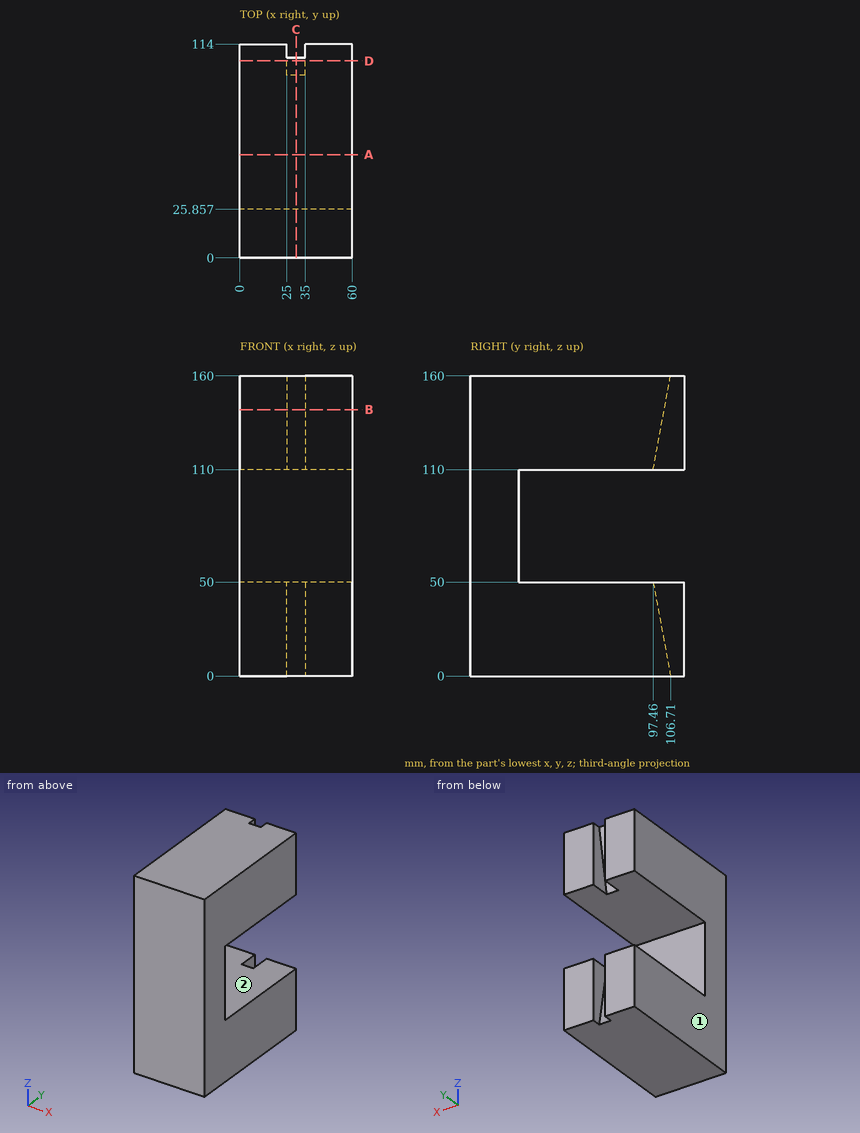
Geometry check sheet. Reference: drawing and pictorial views, mm from the part's lowest x, y, z. A direction names the side the tool comes from. Round coordinates to 2 decimals unless told otherwise and drop trailing zeros. Loops run counter-clockwise (first coordinate to the right, second up) from the corner with the lowest first, then second, coordinate; pieces in that order, holes last. Notation, with made-up numbers: (54, -34) -> (108, -34) arc R31 ccw to (108, -8) -> close; hole circle Ø1 at (5.25, 22.5). An arc over 180 degrees is marked (long way). Answer as a JSON object with one key per item and string values. Group by question number.
Item 1: Cross-section at D-D, the plane y = 105. Record the cut outline in (x, z).
Item 2: Cross-section at C-C, the plane x = 30. Record the cut outline in (y, z).
Item 3: Cross-section at B-B, the plane z = 142. Record the cut outline in (x, y).
Item 4: Depth check by flat-ended pin: pin 1 Ø4 at (x, z) = (44, 57) entering from +Y. Enter the tip coordinate at first touch or a pass-through.
Item 5: Cross-section at A-A, the plane y = 55. Record the cut outline in (x, z).
Item 6: Set-up check for the marked faces 1 and 2: record each of +Z, -Z, +X, -X, +Y, -Y from which the full face is reachable in a straight line by a thin tool's end or side.
Item 7: Thickness scan on line 1 along Z through (x, y) = (32, 85); line 2 along Y through (x, z) = (38, 108); line 3 along X through (y, z) = (105, 27.5). Record the ranges inside material, lowest first.
Determined:
{
 "1": {"outline": "(0, 0) -> (60, 0) -> (60, 50) -> (35, 50) -> (35, 9.24) -> (25, 9.24) -> (25, 50) -> (0, 50) -> close; (0, 110) -> (25, 110) -> (25, 150.76) -> (35, 150.76) -> (35, 110) -> (60, 110) -> (60, 160) -> (0, 160) -> close"},
 "2": {"outline": "(0, 0) -> (106.71, 0) -> (97.46, 50) -> (25.86, 50) -> (25.86, 110) -> (97.46, 110) -> (106.71, 160) -> (0, 160) -> close"},
 "3": {"outline": "(0, 0) -> (60, 0) -> (60, 114) -> (35, 114) -> (35, 103.38) -> (25, 103.38) -> (25, 114) -> (0, 114) -> close"},
 "4": {"pin 1": "stops at y = 25.86"},
 "5": {"outline": "(0, 0) -> (60, 0) -> (60, 50) -> (0, 50) -> close; (0, 110) -> (60, 110) -> (60, 160) -> (0, 160) -> close"},
 "6": {"face 1": "+Z, -Z, -X, +Y, -Y", "face 2": "+X, -X, +Y"},
 "7": {"line 1": "z = 0 to 50, 110 to 160", "line 2": "y = 0 to 25.86", "line 3": "x = 0 to 25, 35 to 60"}
}
